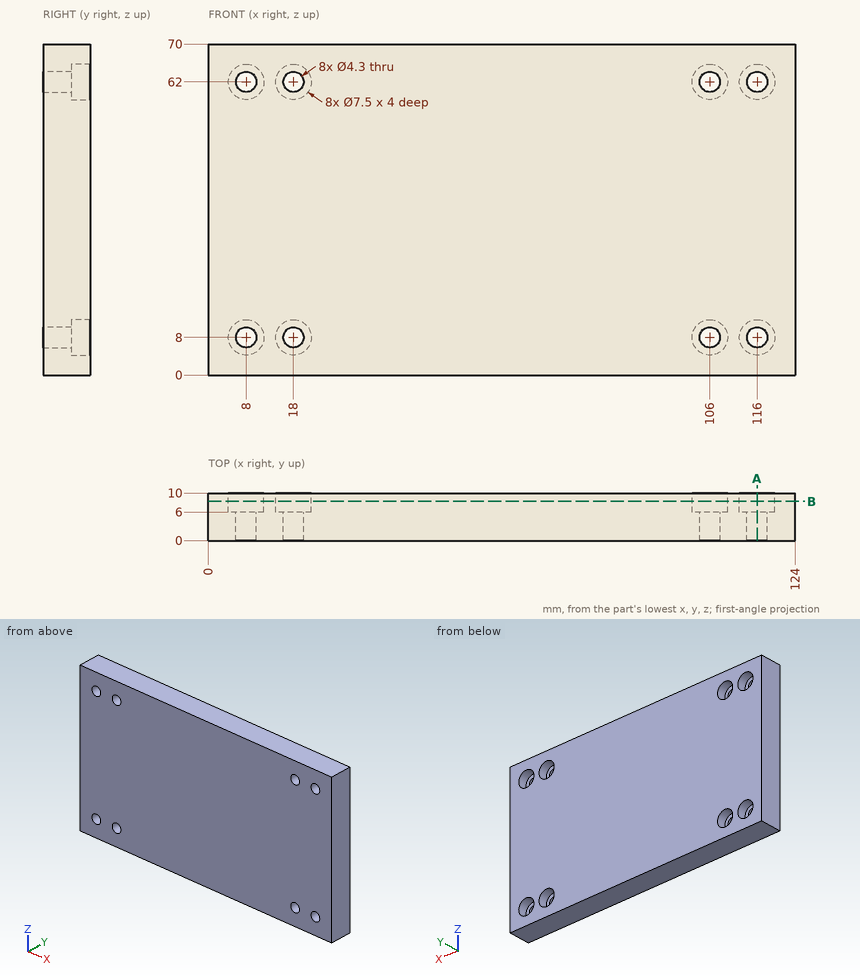
Print and shaded views of the part. All mm, measured from the part's lowest x, y and z. Round coordinates to 2 decimals unless told otherwise and drop trailing zeros. Write each loop counter-clockwise with the first axis right and the second up, starting at its lowest first coordinate (ties: lowest second). Pieces come first, ordered by that corner, then holes. Notation, with made-up numbers: (42.25, -39.75) - (94.25, -39.75) arc R4 cw to (94.25, -35.75) - close; hole circle Ø3 at (79, -9.5). An arc over 180 degrees is marked (long way). Use CSV: the item, a comma, the result in double quotes. Start each with the question number.
Item 1: Drill centre lines: L1, parallel to X at y = 4, z = 62; L2, parallel to X at y = 9, z = 62; L3, parallel to Z at x = 107.5, y = 8.75. Where is each one in solid material? Low to high. Write a range as [from, to].
Item 2: Pin check, flat tips, straight feed: P1, Ø4, axis at x = 116.5, z = 9, coming from the +Y side; P2, Ø3.5, axis at x = 18, z = 8, coming from the +Y side. Stop position of each tip, or through.
Item 3: Band-saw the part on B-B (y = 8.25). State how many separate pieces and enclosed holes the cut face has, and give its area (3 significant figures).
Item 4: Band-saw the part on A-A (x = 116). Write the cut outline in (y, z), and give its area (3 significant figures).
Checked values:
1,L1,"x = [0, 5.85], [10.15, 15.85], [20.15, 103.85], [108.15, 113.85], [118.15, 124]"
1,L2,"x = [0, 4.25], [11.75, 14.25], [21.75, 102.25], [109.75, 112.25], [119.75, 124]"
1,L3,"z = [0, 4.56], [11.44, 58.56], [65.44, 70]"
2,P1,"stops at y = 6"
2,P2,"passes through"
3,separate pieces,"1"
3,enclosed holes,"8"
3,area,"8,330 mm²"
4,outline,"(0, 0) - (10, 0) - (10, 4.25) - (6, 4.25) - (6, 5.85) - (0, 5.85) - close; (0, 10.15) - (6, 10.15) - (6, 11.75) - (10, 11.75) - (10, 58.25) - (6, 58.25) - (6, 59.85) - (0, 59.85) - close; (0, 64.15) - (6, 64.15) - (6, 65.75) - (10, 65.75) - (10, 70) - (0, 70) - close"
4,area,"588 mm²"
